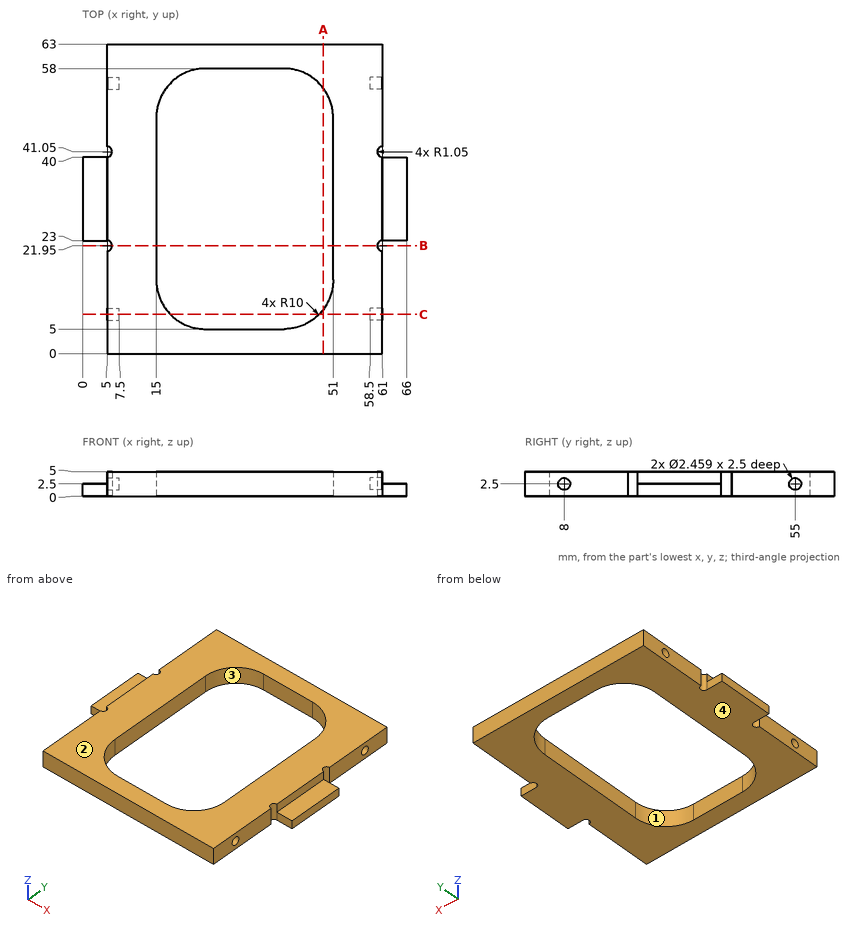
Input: dimensioned drawing with shaded views. Units: mm. Origin: part minimum x, y, z. A direction names the side the tool comes from. Give positions to 0.01 mm unless a question says otherwise; leave off trailing zeros. Loops run counter-clockwise (first coordinate to the right, second up) from the corner with the lowest first, then second, coordinate; pieces in that order, holes last. Notation, with made-up numbers: (9.5, -31) -> (58.5, -31) arc R24 ccw to (58.5, 3) -> close; hole circle Ø10 at (-28, 40). An arc over 180 degrees is marked (long way). Use a Markdown table: item, result. Add a question column.
1) Reachability of the marked faces 3 and 4 from +Z, -Z, +X, -X, +Y, -Y: full face, straight path, thin tool, end or side. Return the list, or none.
2) Section query A-A, the plane x = 49. Return the cut outline in (y, z).
3) First-contact query: pin 1 (2 mm diameter, centred on y = 34.5, z = 4, fed in from -X); pin 2 (0.7 mm diameter, centred on y = 54.5, z = 2.5, fed in from -X); pin 3 (3 mm diameter, centred on x = 2.5, z = 1, fed in from +Y). Flat tips, straight axial feed; report the tip coordinate or a pass-through.
4) Section query B-B, the plane y = 21.95. Return the cut outline in (x, z), then the cut area to 3 significant figures.
5) Section query C-C, the plane y = 8. Return the cut outline in (x, z).
6) Pull-direction query (X, two-part tool) for the marked faces 1 and 2; classes: +X half, -X half, draft (parallel to the pull), parting line (faces both ways), or undercut.
7) Line query: line 1 along Y through (x, z) = (59.3, 2.5); line 2 along X through (y, z) = (25, 4.15); line 3 along Z through (x, y) = (6.9, 8). Output: solid intervals per line, ascending. Write a range as [from, to].
Numbers:
| question | item | result |
|---|---|---|
| 1 | face 3 | +Z, -Z |
| 1 | face 4 | -Z, +X, -X, +Y, -Y |
| 2 | outline | (0, 0) -> (9, 0) -> (9, 5) -> (0, 5) -> close; (54, 0) -> (63, 0) -> (63, 5) -> (54, 5) -> close |
| 3 | pin 1 | stops at x = 5 |
| 3 | pin 2 | stops at x = 7.5 |
| 3 | pin 3 | stops at y = 40 |
| 4 | outline | (6.05, 0) -> (15, 0) -> (15, 5) -> (6.05, 5) -> close; (51, 0) -> (59.95, 0) -> (59.95, 5) -> (51, 5) -> close |
| 4 | area | 89.5 mm2 |
| 5 | outline | (5, 0) -> (17.86, 0) -> (17.86, 5) -> (5, 5) -> (5, 3.73) -> (7.5, 3.73) -> (7.5, 1.27) -> (5, 1.27) -> close; (48.14, 0) -> (61, 0) -> (61, 1.27) -> (58.5, 1.27) -> (58.5, 3.73) -> (61, 3.73) -> (61, 5) -> (48.14, 5) -> close |
| 6 | face 1 | undercut |
| 6 | face 2 | draft |
| 7 | line 1 | y = [0, 6.77], [9.23, 53.77], [56.23, 63] |
| 7 | line 2 | x = [5, 15], [51, 61] |
| 7 | line 3 | z = [0, 1.27], [3.73, 5] |
